```python
from build123d import *

# Parameters (mm, degrees)
SKETCH1_W                = 50
SKETCH1_H                = 30
BOSS_EXTRUDE1_DEPTH      = 6
M5_START                 = -6
M5_CLEARANCE_SLOT1_DEPTH = 12


# Read off the part's stored shape, not the designer's step: M5 Clearance Slot1
with BuildPart() as part:
    # Sketch1 → Boss-Extrude1 (new, symmetric)
    with BuildSketch(Plane.XY):
        Rectangle(SKETCH1_W, SKETCH1_H)
    extrude(amount=BOSS_EXTRUDE1_DEPTH, both=True)

    # M5 Clearance Slot1 outline → M5 Clearance Slot1 (cut)
    with BuildSketch(Plane.XY.offset(M5_START)):
        with BuildLine():
            Line((7.25, 10), (7.25, 3))
            ThreePointArc((7.25, 3), (10, 0.25), (12.75, 3))
            Line((12.75, 3), (12.75, 10))
            ThreePointArc((12.75, 10), (10, 12.75), (7.25, 10))
        make_face()
        with BuildLine():
            Line((-12.75, 10), (-12.75, 3))
            ThreePointArc((-12.75, 3), (-10, 0.25), (-7.25, 3))
            Line((-7.25, 3), (-7.25, 10))
            ThreePointArc((-7.25, 10), (-10, 12.75), (-12.75, 10))
        make_face()
    extrude(amount=M5_CLEARANCE_SLOT1_DEPTH, mode=Mode.SUBTRACT)

    # Sketch5 → M5x0.8 Tapped Hole1 (revolve, cut)
    with BuildSketch(Plane(origin=(15, -15, 0), x_dir=(0, 0, -1), z_dir=(1, 0, 0))):
        Polygon((0, 0), (0, 8.4), (2.1, 7.1381927), (2.1, 0), align=None)
    m5x0_8_tapped_hole1 = revolve(axis=Axis((15, -21.35, 0), (0, 1, 0)), mode=Mode.SUBTRACT)

    # Mirror1: M5x0.8 Tapped Hole1 across plane
    add(m5x0_8_tapped_hole1.mirror(Plane(origin=(0, 0, 0), x_dir=(0, 0, 1), z_dir=(1, 0, 0))), mode=Mode.SUBTRACT)


solid = part.part
```
Work out the finished part from the listing and answer in its coordinate system (mm). A direction names the side the tool comes from. Coordinates: 2 decimals unless noted, no trailing zeros. Loops run counter-clockwise (first coordinate to the right, second up) from the corner with the lowest first, then second, coordinate; pieces in that order, holes last. Notation, with made-up numbers: (0, 86) - (4, 86) arc R4 cw to (4, 90) - close; hole circle Ø6 at (29.25, -13.75). An arc over 180 degrees is marked (long way). Use a Markdown table: item, result.
Item 1: Consider probe 1 along X at (y, z) = (7, 0.5); probe 2 along X at (y, z) = (2.75, 0); probe 3 along Y at (x, z) = (10, -2.25). Determine where each line is inside the solid, lowest interval first. Write a range as from..to.
Evaluation:
| item | result |
|---|---|
| probe 1 | x = -25..-12.75, -7.25..7.25, 12.75..25 |
| probe 2 | x = -25..-12.74, -7.26..7.26, 12.74..25 |
| probe 3 | y = -15..0.25, 12.75..15 |
Item 2: Find section A-A, the plane y = 6.5. Determine the outline of the cut face in (x, z), and give its area (3 significant figures).
Evaluation:
| item | result |
|---|---|
| outline | (-25, -6) - (-12.75, -6) - (-12.75, 6) - (-25, 6) - close; (-7.25, -6) - (7.25, -6) - (7.25, 6) - (-7.25, 6) - close; (12.75, -6) - (25, -6) - (25, 6) - (12.75, 6) - close |
| area | 468 mm2 |
Item 3: Find section D-D, the plane z = 1.25. State how many separate pieces and enclosed holes the cut face has, and give its area (3 significant figures).
Evaluation:
| item | result |
|---|---|
| separate pieces | 1 |
| enclosed holes | 2 |
| area | 1,330 mm2 |
Item 4: Find section B-B, the plane z = 5.25. Determine the outline of the cut face in (x, y).
Evaluation:
| item | result |
|---|---|
| outline | (-25, -15) - (25, -15) - (25, 15) - (-25, 15) - close; hole (-12.75, 3) arc R2.75 ccw to (-7.25, 3) - (-7.25, 10) arc R2.75 ccw to (-12.75, 10) - close; hole (7.25, 3) arc R2.75 ccw to (12.75, 3) - (12.75, 10) arc R2.75 ccw to (7.25, 10) - close |
Item 5: Find section C-C, the plane x = -10. Determine the outline of the cut face in (y, z), and give its area (3 significant figures).
Evaluation:
| item | result |
|---|---|
| outline | (-15, -6) - (0.25, -6) - (0.25, 6) - (-15, 6) - close; (12.75, -6) - (15, -6) - (15, 6) - (12.75, 6) - close |
| area | 210 mm2 |
Item 6: The mould has two halves that part along X. Classify faces 4 (the flat face through (25, 0, 0)), 5 (the flat face through (0, -15, 0)), 6 (the cylindrical face through (12.918, -11.481, 0.273)), 7 (the cylindrical face through (9.94, 0.25, -0.08)): +X half, -X half, draft (parallel to the pull), parting line (faces both ways), or undercut.
Evaluation:
| item | result |
|---|---|
| face 4 | +X half |
| face 5 | draft |
| face 6 | undercut |
| face 7 | undercut |
Item 7: For faces 1 (the cylindrical face through (-12.918, -11.481, 0.273)), 2 (the flat face through (-7.25, 6, 0)), 3 (the flat face through (0, 15, 0)), determine the directions among +Z, -Z, +X, -X, +Y, -Y from which every point of the face is accessible in a straight line to the end or side of a thin tool.
Evaluation:
| item | result |
|---|---|
| face 1 | -Y |
| face 2 | +Z, -Z |
| face 3 | +Z, -Z, +X, -X, +Y |
